```python
from build123d import *

# Parameters (mm, degrees)
F0_R        = 0.85
F1_DEPTH    = 1
F2_T1_DEPTH = 1
F3_R        = 3


# Not quite as in the source:
# - a fillet or chamfer that OpenCascade refuses, or shapes differently, is made with other operations: its cross-section is extruded or revolved along the edge and cut away or added


with BuildPart() as f1:
    # F0 (on Front) → F1 (new body)
    with BuildSketch(Plane.XZ):
        with BuildLine():
            ThreePointArc((-0.85, -7.0992957397), (0, 7.15), (0.85, -7.0992957397))
            Line((0.85, -7.0992957397), (0.85, -10.7163426597))
            ThreePointArc((0.85, -10.7163426597), (3.1412802118, -10.2808004859), (5.2846966911, -9.3613290127))
            Line((5.2846966911, -9.3613290127), (4.5, -7.6785415282))
            ThreePointArc((4.5, -7.6785415282), (0, 9.3500403242), (-4.5, -7.6785415282))
            Line((-4.5, -7.6785415282), (-5.2846966911, -9.3613290127))
            ThreePointArc((-5.2846966911, -9.3613290127), (-3.1412802118, -10.2808004859), (-0.85, -10.7163426597))
            Line((-0.85, -10.7163426597), (-0.85, -7.0992957397))
        make_face()
        with Locations((-2.6762816156, -8.4880808617)):
            Circle(F0_R, mode=Mode.SUBTRACT)
        with Locations((2.6762816156, -8.4880808617)):
            Circle(F0_R, mode=Mode.SUBTRACT)
    extrude(amount=F1_DEPTH)

    # F2: fillet of radius 3 on 2 edges, made by hand

    # F2_s2 → F2_t1 (join)
    with BuildSketch(Plane.XZ):
        with BuildLine():
            ThreePointArc((-6.170677683, -6.4591691909), (-5.3337110531, -7.7899747588), (-5.2846966911, -9.3613290127))
            Line((-5.2846966911, -9.3613290127), (-4.5, -7.6785415282))
            ThreePointArc((-4.5, -7.6785415282), (-5.3700612452, -7.1164289704), (-6.170677683, -6.4591691909))
        make_face()
        with BuildLine():
            ThreePointArc((5.2846966911, -9.3613290127), (5.3337110531, -7.7899747588), (6.170677683, -6.4591691909))
            ThreePointArc((6.170677683, -6.4591691909), (5.3700612452, -7.1164289704), (4.5, -7.6785415282))
            Line((4.5, -7.6785415282), (5.2846966911, -9.3613290127))
        make_face()
    extrude(amount=F2_T1_DEPTH)

    # F3
    f3_edges = [f1.edges().sort_by_distance(p)[0] for p in [
        (-5.284697, -0.5, -9.361329),
        (5.284697, -0.5, -9.361329),
    ]]
    fillet(f3_edges, radius=F3_R)


solid = f1.part
```
Part model, mm, in its own coordinate system. A direction names the side the tool comes from. Round coordinates to 2 decimals unless told otherwise and drop trailing zeros. Write each loop counter-clockwise with the first axis right and the second up, starting at its lowest first coordinate (ties: lowest second). Pieces come first, ordered by that corner, then holes.
Item 1: Cut at C-C, the plane x = 0. Give the cut face in (y, z), plus the area to 3 significant figures.
Results:
outline: (-1, 7.15) - (0, 7.15) - (0, 9.35) - (-1, 9.35) - close
area: 2.20 mm2
Item 2: Two-plate mould, pull along X, no slides. Class faces 1 (the cylindrical face through (-5.61, -0.49, -7.16)), 2 (the flat face through (7, -1, -3)), 3 (the cylindrical face through (3.07, -0.49, -9.24)): +X half, -X half, draft (parallel to the pull), parting line (faces both ways), or undercut.
Results:
face 1: -X half
face 2: draft
face 3: undercut
Item 3: Probe L1, parallel to X at y = -0.75, z = -0.5; L2, parallel to X at y = -0.15, z = 2.25; L3, parallel to Z at x = -2.75, y = -0.4 (3 decimals). List the from-to ranges inside material, lowest first.
Results:
L1: x = -9.08 to -7.13, 7.13 to 9.08
L2: x = -8.88 to -6.79, 6.79 to 8.88
L3: z = -10.392 to -9.335, -7.641 to -6.6, 6.6 to 8.925
Item 4: Cut at D-D, the plane y = -0.7. Count the separate pieces of the cut face and the enclosed holes in it, plus the area to 3 significant figures.
Results:
separate pieces: 1
enclosed holes: 2
area: 109 mm2
Item 5: Cut at A-A, the plane z = 0.5. Give the cut face in (x, y), plus the area to 3 significant figures.
Results:
outline: (-9.11, -1) - (-7.13, -1) - (-7.13, 0) - (-9.11, 0) - close; (7.13, -1) - (9.11, -1) - (9.11, 0) - (7.13, 0) - close
area: 3.95 mm2
Item 6: Drop flat-ended pins along their axis: pin 1 Ø1.5 at (x, z) = (-2.68, -8.49) entering from -Y; pin 2 Ø0.5 at (y, z) = (-0.5, -8.5) entering from +X. Give the stop position or say it passes through.
Results:
pin 1: passes through
pin 2: stops at x = 5.21
Item 7: Which spindle directions (+Z, -Z, +X, -X, +Y, -Y) get a long thin tool onto all of the face, cutting with end or side? Do faces 4 (the flat face through (-0.85, -0.5, -8.9)), 5 (the cylindrical face through (-0.302, -0.493, 7.144)). Say none if no direction does.
Results:
face 4: -Z, +Y, -Y
face 5: +Y, -Y
Item 8: Cut at B-B, the plane z = -3.5. Give the cut face in (x, y).
Results:
outline: (-8.31, -1) - (-6.23, -1) - (-6.23, 0) - (-8.31, 0) - close; (6.23, -1) - (8.31, -1) - (8.31, 0) - (6.23, 0) - close
